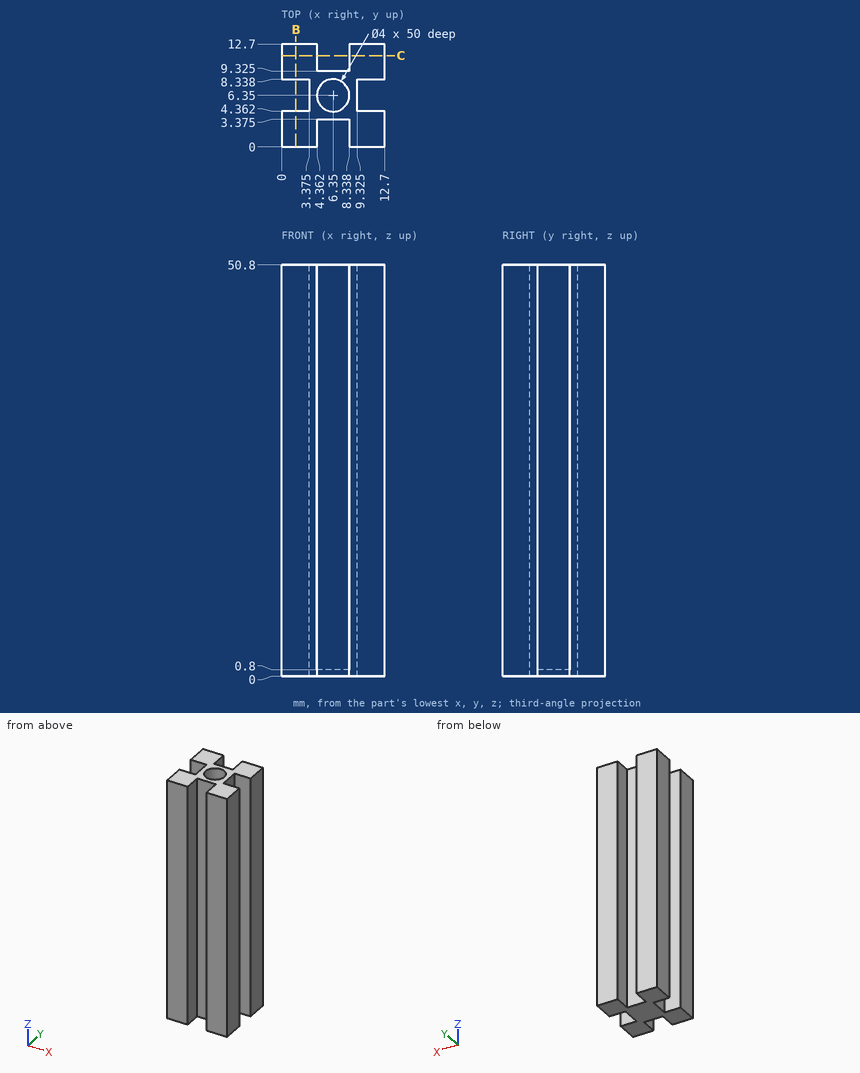
Verification items for this drawing (mm, ordinates from the low corner). Coordinates: 2 decimals unless noted, no trailing zeros. Order: outer loops, then holes, each group sorted by start corner. A loop starts at its lowest first (then second) coordinate and runs counter-clockwise, first axis right, second up. Notation, with made-up numbers: (28.25, 24) -> (68.25, 24) arc R24 cw to (68.25, 60) -> close; hole circle Ø9 at (31, 83). An arc over 180 degrees is marked (long way). Put each result on its own line as item: value. Start each with the question number.
1. Cross-section at B-B, the plane x = 1.75. Record the boundary of the cut face in (y, z), then the cut area to 3 significant figures.
2. Material ranges on L1, parallel to X at y = 1.25, z = 26.5; L2, parallel to X at y = 6.5, z = 26.5 (1 decimal), recorded low to high. Write a range as [from, to].
3. Go/stop test with flat-tipped pins: pin 1 Ø2 at (y, z) = (7, 28.5) entering from -X (1 decimal); pin 2 Ø2 at (x, z) = (5.5, 37.5) entering from +Y (1 decimal); pin 3 Ø3.5 at (x, y) = (6.35, 6.35) entering from +Z. Record where each tip stops, or that it passes through.
Computed:
1. outline: (0, 0) -> (4.36, 0) -> (4.36, 50.8) -> (0, 50.8) -> close; (8.34, 0) -> (12.7, 0) -> (12.7, 50.8) -> (8.34, 50.8) -> close
1. area: 443 mm2
2. L1: [0, 4.36], [8.34, 12.7]
2. L2: [3.4, 4.4], [8.3, 9.3]
3. pin 1: x = 3.4
3. pin 2: y = 9.3
3. pin 3: z = 0.8
